from build123d import *

# Parameters (mm, degrees)
SKETCH1_W   = 300
SKETCH1_H   = 70
WALL_DEPTH  = 6
SKETCH2_W   = 6
SKETCH2_H   = 40
SKETCH2_H_2 = 20
MOUNT_DEPTH = 309.116860947
SKETCH3_R   = 17.5
LITE_DEPTH  = 309.116860947
FILLET_2_R  = 1


with BuildPart() as part:
    # Sketch1 → wall (new body)
    with BuildSketch(Plane(origin=(0, 0, 0), x_dir=(0, 0, -1), z_dir=(1, 0, 0))):
        with Locations((150, 35)):
            Rectangle(SKETCH1_W, SKETCH1_H)
    extrude(amount=WALL_DEPTH)

    # Sketch2 → mount (cut, through all)
    with BuildSketch(Plane(origin=(6, 0, 0), x_dir=(0, 0, -1), z_dir=(1, 0, 0))):
        with Locations((177, 35)):
            Rectangle(SKETCH2_W, SKETCH2_H)
        with Locations((297, 35)):
            Rectangle(SKETCH2_W, SKETCH2_H_2)
        with Locations((3, 35)):
            Rectangle(SKETCH2_W, SKETCH2_H_2)
    extrude(amount=-MOUNT_DEPTH, mode=Mode.SUBTRACT)

    # Sketch3 → lite (cut, through all)
    with BuildSketch(Plane(origin=(6, 0, 0), x_dir=(0, 0, -1), z_dir=(1, 0, 0))):
        with Locations((50, 35)):
            Circle(SKETCH3_R)
        with Locations((115, 35)):
            Circle(SKETCH3_R)
        with Locations((240, 35)):
            Circle(SKETCH3_R)
    extrude(amount=-LITE_DEPTH, mode=Mode.SUBTRACT)

    # fillet 2
    fillet_2_edges = [part.edges().sort_by_distance(p)[0] for p in [
        (3, 70, 0),
        (3, 70, -300),
        (3, 0, -300),
        (3, 0, 0),
    ]]
    fillet(fillet_2_edges, radius=FILLET_2_R)


solid = part.part
CAD build for the part. Positions are in the model's coordinates, mm. A direction names the side the tool comes from. Give positions to 0.01 mm unless a question says otherwise; leave off trailing zeros. Write each loop counter-clockwise with the first axis right and the second up, starting at its lowest first coordinate (ties: lowest second). Pieces come first, ordered by that corner, then holes. Notation, with made-up numbers: M 24.5,23 L 70.5,23 A13 cw 70.5,44 Z; hole C -12,35.5 d2. An arc over 180 degrees is marked long. Put each result on its own line as item: value. Start each with the question number.
(1) Mould opens along Z. For faces 5 (the face through (3, 35, -294)), 6 (the face through (3.04, 40.26, -131.69)), 7 (the face through (3, 45, -297)) say: +Z half, -Z half, draft (parallel to the pull), parting line (faces both ways), or undercut.
(2) Band-saw the part on D-D, the plane y = 22.5. Write the cut outline in (x, z).
(3) Probe L1, parallel to Y at x = 1.15, z = -178.5; L2, parallel to Z at x = 4.55, y = 39.5; L3, parallel to Y at x = 4.5, z = -115. List the from-to ranges inside material, lowest first.
(4) Band-saw the part on A-A, the plane z = -240. Write the cut outline in (x, y), and give its area (3 significant figures).
(5) Which spindle directions (+Z, -Z, +X, -X, +Y, -Y) get a long thin tool onto all of the face, cutting with end or side? Do faces 1 (the face through (3, 55, -177)), 2 (the face through (3, 25, -3)), 3 (the face through (3, 25, -297)), 4 (the face through (0, 35, -148)). Say none if no direction does.
(6) Band-saw the part on C-C, the plane x = 1.5. Write the cut outline in (y, z).
(7) Flat gauge pins, fed straight in: pin 1 Ø21 at (y, z) = (35, -115) entering from -X; pin 2 Ø1.8 at (x, y) = (2, 44) entering from +Z. Where does each tip first touch, or does it go through?
(8) Band-saw the part on B-B, the plane y = 35. Write the cut outline in (x, z).
Response values:
1. face 5: -Z half
1. face 6: undercut
1. face 7: draft
2. outline: M 0,-300 L 6,-300 L 6,-252.25 L 0,-252.25 Z; M 0,-227.75 L 6,-227.75 L 6,-180 L 0,-180 Z; M 0,-174 L 6,-174 L 6,-127.25 L 0,-127.25 Z; M 0,-102.75 L 6,-102.75 L 6,-62.25 L 0,-62.25 Z; M 0,-37.75 L 6,-37.75 L 6,0 L 0,0 Z
3. L1: y = 0 to 15, 55 to 70
3. L2: z = -294 to -256.91, -223.09 to -180, -174 to -131.91, -98.09 to -66.91, -33.09 to -6
3. L3: y = 0 to 17.5, 52.5 to 70
4. outline: M 0,0 L 6,0 L 6,17.5 L 0,17.5 Z; M 0,52.5 L 6,52.5 L 6,70 L 0,70 Z
4. area: 210 mm2
5. face 1: +X, -X
5. face 2: +Z, +X, -X
5. face 3: -Z, +X, -X
5. face 4: +Z, -Z, -X, +Y, -Y
6. outline: M 0,-299 A1 ccw 1,-300 L 25,-300 L 25,-294 L 45,-294 L 45,-300 L 69,-300 A1 ccw 70,-299 L 70,-1 A1 ccw 69,0 L 45,0 L 45,-6 L 25,-6 L 25,0 L 1,0 A1 ccw 0,-1 Z; hole M 15,-180 L 55,-180 L 55,-174 L 15,-174 Z; hole C 35,-240 d35; hole C 35,-115 d35; hole C 35,-50 d35
7. pin 1: passes through
7. pin 2: stops at z = -6
8. outline: M 0,-294 L 6,-294 L 6,-257.5 L 0,-257.5 Z; M 0,-222.5 L 6,-222.5 L 6,-180 L 0,-180 Z; M 0,-174 L 6,-174 L 6,-132.5 L 0,-132.5 Z; M 0,-97.5 L 6,-97.5 L 6,-67.5 L 0,-67.5 Z; M 0,-32.5 L 6,-32.5 L 6,-6 L 0,-6 Z
